```python
from build123d import *

# Parameters (mm, degrees)
F0_R     = 203.2
F0_R_2   = 192.8876
F1_DEPTH = 968.375
F2_W     = 228.6
F2_H     = 514.2992
F3_DEPTH = 215.9


with BuildPart() as f1:
    # F0 (on Top) → F1 (new body)
    with BuildSketch(Plane.XY):
        Circle(F0_R)
        Circle(F0_R_2, mode=Mode.SUBTRACT)
    extrude(amount=F1_DEPTH)

    # F2 (on Front) → F3 (cut, symmetric)
    with BuildSketch(Plane.XZ):
        with Locations((0, 629.2818784714)):
            Rectangle(F2_W, F2_H)
    extrude(amount=F3_DEPTH, both=True, mode=Mode.SUBTRACT)


solid = f1.part
```
Design review of the part built by this model. Coordinates are the model's own, in mm. Coordinates: 2 decimals unless noted, no trailing zeros. Loops run counter-clockwise (first coordinate to the right, second up) from the corner with the lowest first, then second, coordinate; pieces in that order, holes last. Notation, with made-up numbers: (25, 58) -> (61, 58) arc R27 ccw to (61, 75) -> close; hole circle Ø4 at (-37.75, 79.25). An arc over 180 degrees is marked (long way). Answer as a JSON object with one key per item and string values.
Q1. To check wall thickness, follow L1, parallel to Y at x = -114, z = 929.5; L2, parallel to Y at x = 0, z = 356.5; L3, parallel to X at y = -71.5, z = 916.5. State the ranges of each line that lie inside material, in increasing order.
Answer block:
{"L1": "y = -168.21 to -155.59, 155.59 to 168.21", "L2": "y = -203.2 to -192.89, 192.89 to 203.2", "L3": "x = -190.21 to -179.15, 179.15 to 190.21"}
Q2. Clearance check with flat-ended pins moving along their axes: pin 1 Ø8 at (y, z) = (-48.5, 213) entering from -X; pin 2 Ø5 at (y, z) = (-71.5, 576.5) entering from +X; pin 3 Ø10 at (y, z) = (-161.5, 511) entering from -X. State where each tip first meets the part, or that it passes through.
Answer block:
{"pin 1": "stops at x = -198.27", "pin 2": "stops at x = 191.13", "pin 3": "stops at x = -129.61"}
Q3. The part is to be moulded in two halves that separate along Z. For faces 1 (the flat face through (-1, 195, 372.132)), 2 (the flat face through (180, -74, 968.375)), 3 (the flat face through (180, -74, 0)), say which applies: +Z half, -Z half, draft (parallel to the pull), parting line (faces both ways), or undercut.
Answer block:
{"face 1": "undercut", "face 2": "+Z half", "face 3": "-Z half"}
Q4. Take a section at B-B on x = 0. Give the boundary of the cut face in (y, z) (3 decimals).
Answer block:
{"outline": "(-203.2, 0) -> (-192.888, 0) -> (-192.888, 372.132) -> (-203.2, 372.132) -> close; (-203.2, 886.431) -> (-192.888, 886.431) -> (-192.888, 968.375) -> (-203.2, 968.375) -> close; (192.888, 0) -> (203.2, 0) -> (203.2, 372.132) -> (192.888, 372.132) -> close; (192.888, 886.431) -> (203.2, 886.431) -> (203.2, 968.375) -> (192.888, 968.375) -> close"}
Q5. Take a section at A-A on y = 0. Give the boundary of the cut face in (x, z) (3 decimals).
Answer block:
{"outline": "(-203.2, 0) -> (-192.888, 0) -> (-192.888, 968.375) -> (-203.2, 968.375) -> close; (192.888, 0) -> (203.2, 0) -> (203.2, 968.375) -> (192.888, 968.375) -> close"}
Q6. Take a section at D-D on z = 906.5. Give the boundary of the cut face in (x, y).
Answer block:
{"outline": "circle Ø406.4 at (0, 0); hole circle Ø385.78 at (0, 0)"}
Q7. Take a section at C-C on x = 126.5. Give the boundary of the cut face in (y, z) (3 decimals).
Answer block:
{"outline": "(-159.022, 0) -> (-145.614, 0) -> (-145.614, 968.375) -> (-159.022, 968.375) -> close; (145.614, 0) -> (159.022, 0) -> (159.022, 968.375) -> (145.614, 968.375) -> close"}
